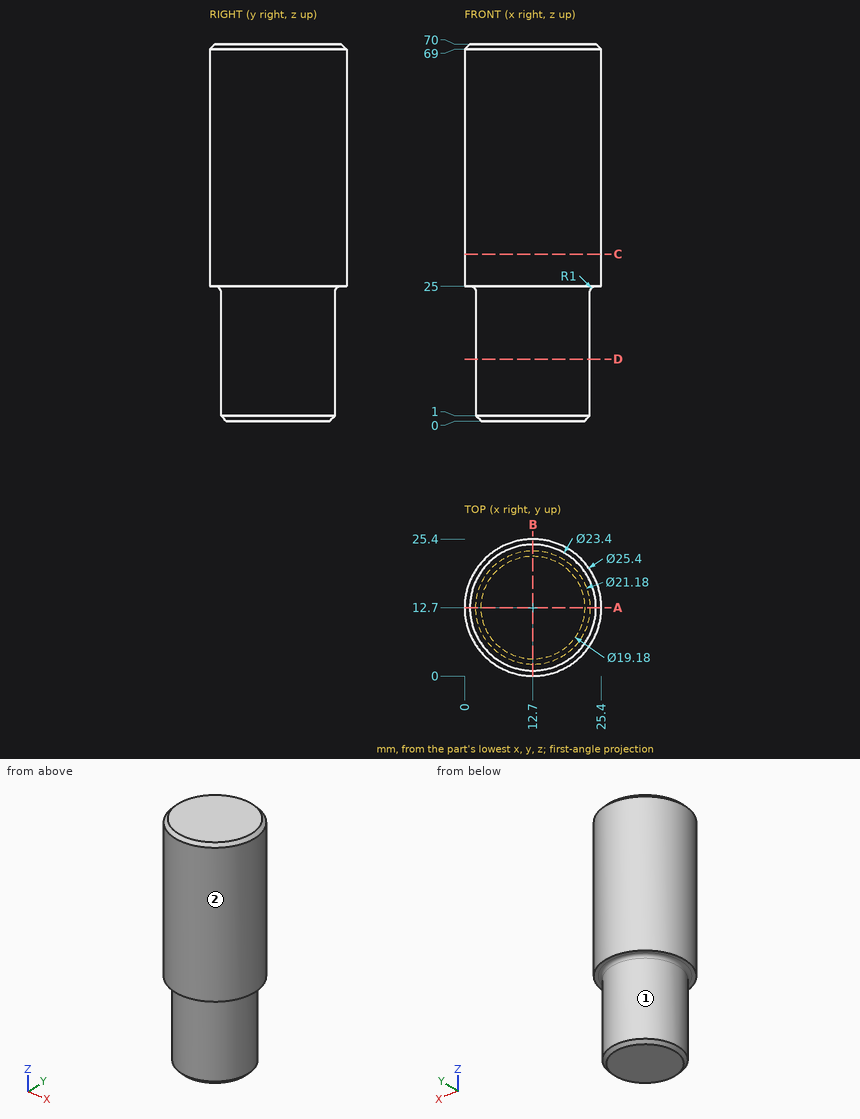
Here's the drawing with two shaded views (mm, measured from the low corner). I have some questions. A direction names the side the tool comes from. Give positions to 0.01 mm unless a question says otherwise; leave off trailing zeros. Order: outer loops, then holes, each group sorted by start corner. A loop starts at its lowest first (then second) coordinate and runs counter-clockwise, first axis right, second up. Notation, with made-up numbers: (4.5, 2) - (25.5, 2) arc R21 ccw to (25.5, 19) - close; hole circle Ø2 at (1, 67). An arc over 180 degrees is marked (long way). Use a Markdown table: item, result. Add a question column.
Q1. If we section it at C-C on z = 31: Write out the boundary of the cut face in (x, y), plus the area to 3 significant figures.
Q2. If we section it at D-D on z = 11.5: Write out the boundary of the cut face in (x, y), plus the area to 3 significant figures.
Q3. If we section it at A-A on y = 12.7: Write out the boundary of the cut face in (x, z).
Q4. I'm going to push flat-ended pins straight in: pin 1 (10 mm diameter, centred on y = 22.5, z = 12, fed in from -X); pin 2 (2 mm diameter, centred on x = 6, z = 33, fed in from -Y); pin 3 (6 mm diameter, centred on x = 9.5, z = 26, fed in from +Y); pin 4 (8 mm diameter, centred on y = 8.5, z = 17.5, fed in from -X). Where does each tip first touch, or does it pass through?
Q5. Please list where these lines run through material, in increasing order: line 1 along X through (y, z) = (7.5, 56); line 2 along Y through (x, z) = (13.25, 43); line 3 along Y through (x, z) = (16.5, 36.5).
Q6. On a 3-axis mill with a long thin cutter (end or side, diameter ignored), from which of +Z, -Z, +X, -X, +Y, -Y can I reach the whole of each face in a straight line? I mean the marked faces 1 and 2. Say none if no direction works.
Answers follow:
| question | item | result |
|---|---|---|
| 1 | outline | circle Ø25.4 at (12.7, 12.7) |
| 1 | area | 507 mm^2 |
| 2 | outline | circle Ø21.18 at (12.7, 12.7) |
| 2 | area | 352 mm^2 |
| 3 | outline | (0, 25) - (1.11, 25) arc R1 cw to (2.11, 24) - (2.11, 1) - (3.11, 0) - (22.29, 0) - (23.29, 1) - (23.29, 24) arc R1 cw to (24.29, 25) - (25.4, 25) - (25.4, 69) - (24.4, 70) - (1, 70) - (0, 69) - close |
| 4 | pin 1 | stops at x = 3.26 |
| 4 | pin 2 | stops at y = 1.35 |
| 4 | pin 3 | stops at y = 25.4 |
| 4 | pin 4 | stops at x = 2.11 |
| 5 | line 1 | x = 1.11 to 24.29 |
| 5 | line 2 | y = 0.01 to 25.39 |
| 5 | line 3 | y = 0.58 to 24.82 |
| 6 | face 1 | -Z |
| 6 | face 2 | +Z, -Z |
